Could you check a few things on this drawing? It's one solid part, dimensions in mm from its lowest x, y, z. A direction names the side the tool comes from. Round coordinates to 2 decimals unless told otherwise and drop trailing zeros. Loops run counter-clockwise (first coordinate to the right, second up) from the corner with the lowest first, then second, coordinate; pieces in that order, holes last. Notation, with made-up numbers: (-2.5, 81) -> (39.5, 81) arc R12 ccw to (39.5, 89) -> close; hole circle Ø10 at (44.25, 18.5). An arc over 180 degrees is marked (long way). Write each question's results on one line, items separated by ' | '.
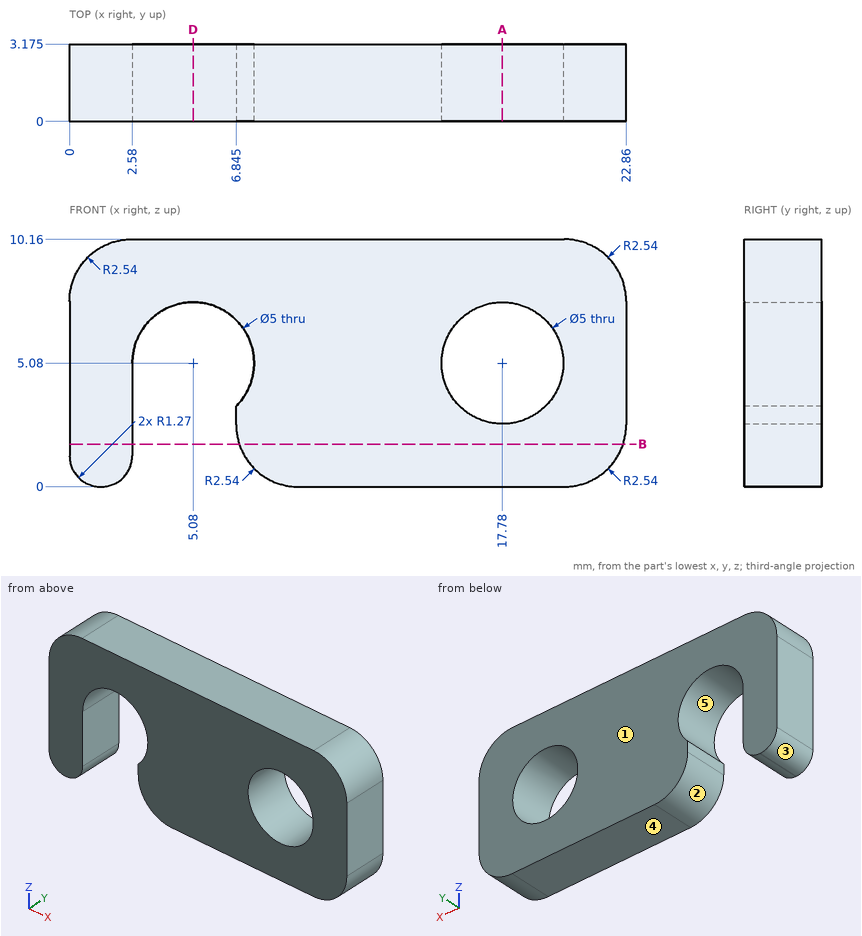
1) I want a section at D-D, the plane x = 5.08. Write out the boundary of the cut face in (y, z) (1 decimal).
Model answer:
outline: (0, 7.6) -> (3.2, 7.6) -> (3.2, 10.2) -> (0, 10.2) -> close
2) I'm going to push a flat-ended pin straight in: pin 1 (1.5 mm diameter, centred on y = 1, z = 1.5, fed in from +X). Where does the tip first touch, or does it pass through?
Model answer:
pin 1: stops at x = 22.84
3) If we mould it in two halves opening along X, with no side actions, what happens to the marked faces 3, 4 and 5? For each: released by +X, released by -X, zero draft, split by the parting line, or undercut.
Model answer:
face 3: released by -X | face 4: zero draft | face 5: undercut
4) I want a section at A-A, the plane x = 17.78. Write out the boundary of the cut face in (y, z) (1 decimal).
Model answer:
outline: (0, 0) -> (3.2, 0) -> (3.2, 2.6) -> (0, 2.6) -> close; (0, 7.6) -> (3.2, 7.6) -> (3.2, 10.2) -> (0, 10.2) -> close
5) For the marked faces 1 and 2, which set-ups out of +Z, -Z, +X, -X, +Y, -Y let a thin tool reach every point of the face, with its end or its side?
Model answer:
face 1: +Z, -Z, +X, -X, +Y | face 2: -Z, +Y, -Y
6) I want a section at B-B, the plane z = 1.75. Write out the boundary of the cut face in (x, y) (1 decimal).
Model answer:
outline: (0, 0) -> (2.6, 0) -> (2.6, 3.2) -> (0, 3.2) -> close; (7, 0) -> (22.7, 0) -> (22.7, 3.2) -> (7, 3.2) -> close
7) I need wall thicknesses on line 1 (X direction, y = 1.8, z = 5.08); line 2 (X direction, y = 0.6, z = 7.25) (1 decimal); line 3 (Z direction, x = 17.78, y = 1.05). Which ranges of each line are inside material? Lowest first, please.
Model answer:
line 1: x = 0 to 2.58, 7.58 to 15.28, 20.28 to 22.86 | line 2: x = 0 to 3.8, 6.3 to 16.5, 19 to 22.9 | line 3: z = 0 to 2.58, 7.58 to 10.16
